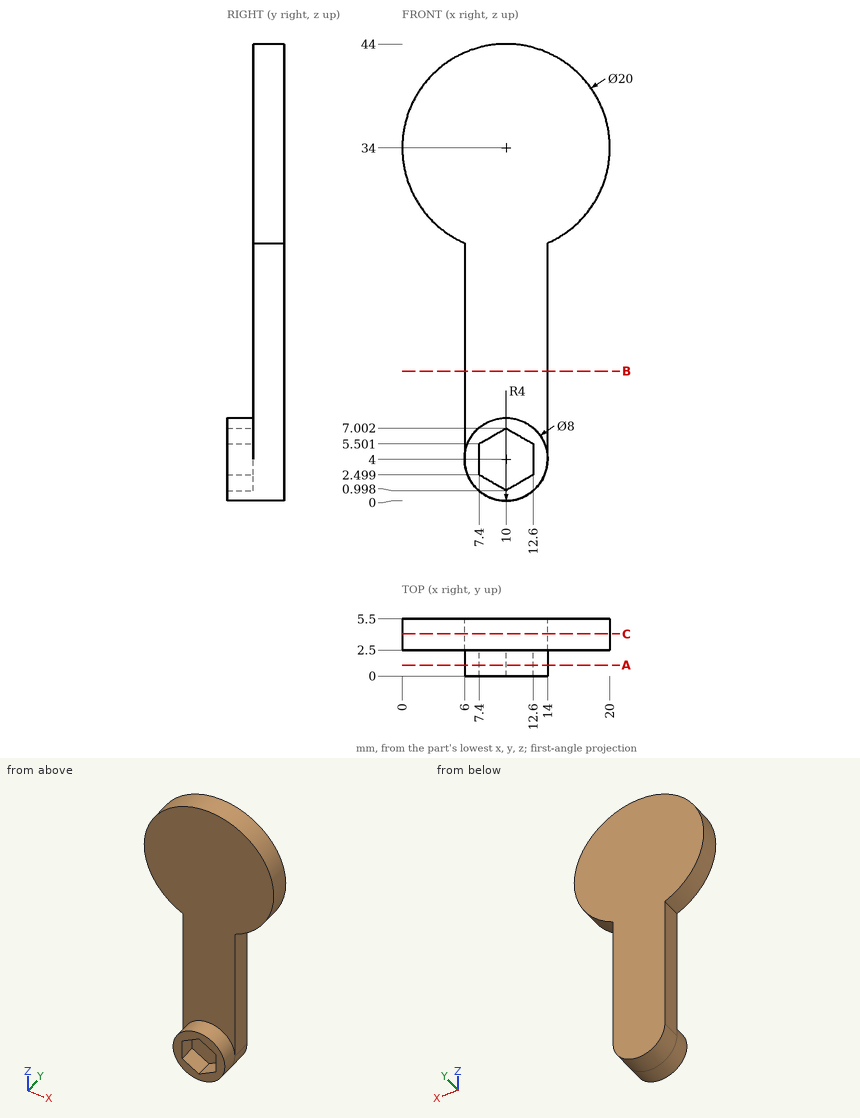
Here's the drawing with two shaded views (mm, measured from the low corner). I have some questions. Coordinates: 2 decimals unless noted, no trailing zeros. Write each loop counter-clockwise with the first axis right and the second up, starting at its lowest first coordinate (ties: lowest second). Pieces come first, ordered by that corner, then holes.
Item 1: I want a section at C-C on y = 4.05. Write out the boundary of the cut face in (x, z) (1 decimal).
Item 2: Will these pins go through, and if not, where does the flat tip stop? pin 1 (10 mm diameter, centred on x = 13, z = 14.5, fed in from -Y); pin 2 (1.5 mm diameter, centred on x = 12.5, y = 4.5, fed in from -Z); pin 3 (0.8 mm diameter, centred on y = 1.5, z = 4.5, fed in from -X).
Item 3: If I drill on line 1 (Y direction, x = 11.75, z = 17); line 2 (X direction, y = 2.1, z = 4); line 3 (Z direction, x = 9.25, y = 2.35), over which ranges is the centre line in solid material (lowest first)?
Item 4: I want a section at B-B on z = 12.5. Write out the boundary of the cut face in (x, y).
Item 5: I want a section at A-A on y = 1.05. Write out the boundary of the cut face in (x, z).
Findings below:
1. outline: (6, 4) arc R4 ccw to (14, 4) - (14, 24.8) arc R10 ccw (long way) to (6, 24.8) - close
2. pin 1: stops at y = 2.5
2. pin 2: stops at z = 0.4
2. pin 3: stops at x = 6
3. line 1: y = 2.5 to 5.5
3. line 2: x = 6 to 7.4, 12.6 to 14
3. line 3: z = 0.07 to 1.43, 6.57 to 7.93
4. outline: (6, 2.5) - (14, 2.5) - (14, 5.5) - (6, 5.5) - close
5. outline: circle Ø8 at (10, 4); hole (7.4, 2.5) - (10, 1) - (12.6, 2.5) - (12.6, 5.5) - (10, 7) - (7.4, 5.5) - close
